from build123d import *

# Parameters (mm, degrees)
SKETCH1_R                        = 23.01875
SKETCH1_R_2                      = 11.1125
BOSS_EXTRUDE1_DEPTH              = 76.2
SKETCH2_R                        = 16.66875
SKETCH2_R_2                      = 11.1125
BOSS_EXTRUDE2_DEPTH              = 31.75
CUT_EXTRUDE1_DEPTH               = 44.45
F_10_0_1935_DIAMETER_HOLE1_D     = 4.9149
F_10_0_1935_DIAMETER_HOLE1_DEPTH = 3.175
F_10_0_1935_DIAMETER_HOLE1_TIP   = 1.476584928


with BuildPart() as part:
    # Sketch1 → Boss-Extrude1 (new body)
    with BuildSketch(Plane(origin=(0, 0, 0), x_dir=(1, 0, 0), z_dir=(0, 1, 0))):
        Circle(SKETCH1_R)
        Circle(SKETCH1_R_2, mode=Mode.SUBTRACT)
    extrude(amount=BOSS_EXTRUDE1_DEPTH)

    # Sketch2 → Boss-Extrude2 (add)
    with BuildSketch(Plane(origin=(0, 76.2, 0), x_dir=(1, 0, 0), z_dir=(0, 1, 0))):
        Circle(SKETCH2_R)
        Circle(SKETCH2_R_2, mode=Mode.SUBTRACT)
    extrude(amount=BOSS_EXTRUDE2_DEPTH)

    # Sketch3 → Cut-Revolve1 (revolve, cut)
    with BuildSketch(Plane(origin=(0, 0, 0), x_dir=(0, 0, -1), z_dir=(1, 0, 0))):
        Polygon((16.66875, 107.95), (16.66875, 100.57660721), (11.1125, 107.95), align=None)
    revolve(axis=Axis((0, 107.95, 0), (0, 1, 0)), mode=Mode.SUBTRACT)

    # Sketch4 → Cut-Extrude1 (cut)
    with BuildSketch(Plane(origin=(0, 76.2, 0), x_dir=(1, 0, 0), z_dir=(0, 1, 0))):
        with BuildLine():
            Line((8.400260413, -21.43125), (-8.400260413, -21.43125))
            ThreePointArc((-8.400260413, -21.43125), (0, -23.01875), (8.400260413, -21.43125))
        make_face()
    extrude(amount=-CUT_EXTRUDE1_DEPTH, mode=Mode.SUBTRACT)

    # Sketch8 → Cut-Revolve4 (revolve, cut)
    with BuildSketch(Plane.XY):
        with BuildLine():
            Line((0, 0), (-3.369464108, 0))
            ThreePointArc((-3.369464108, 0), (-13.321537524, 0.798864496), (-23.01875, 3.175))
            Line((-23.01875, 3.175), (-23.01875, -4.469484217))
            Line((-23.01875, -4.469484217), (0, -4.469484217))
            Line((0, -4.469484217), (0, 0))
        make_face()
    revolve(axis=Axis((0, 0, 0), (0, 1, 0)), mode=Mode.SUBTRACT)

    # 10 _0.1935_ Diameter Hole1
    with Locations(Plane.XY.offset(21.43125)):
        with Locations((0, 68.2625), (0, 39.6875)):
            Hole(F_10_0_1935_DIAMETER_HOLE1_D / 2, depth=F_10_0_1935_DIAMETER_HOLE1_DEPTH)
            with Locations((0, 0, -(F_10_0_1935_DIAMETER_HOLE1_DEPTH + F_10_0_1935_DIAMETER_HOLE1_TIP / 2))):  # 118° drill point
                Cone(0, F_10_0_1935_DIAMETER_HOLE1_D / 2, F_10_0_1935_DIAMETER_HOLE1_TIP, mode=Mode.SUBTRACT)


solid = part.part
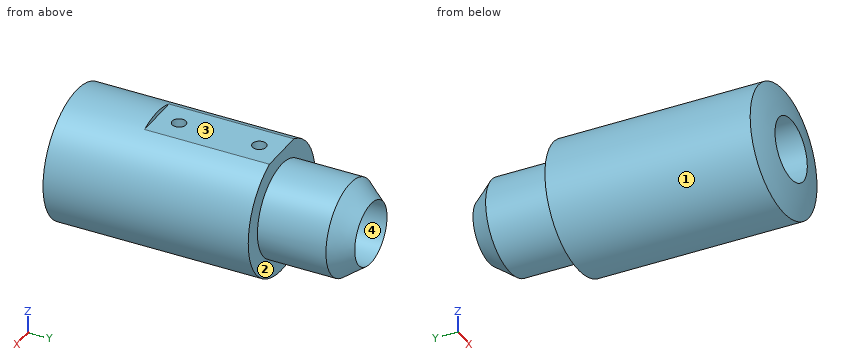
Can you work these out from the model? Positions are in its coordinate system, mm. Face numbers are marked on the shaded views. Give positions to 0.01 mm unless a question says otherwise; leave off trailing zeros. Loops run counter-clockwise (first coordinate to the right, second up) from the corner with the lowest first, then second, coordinate; pieces in that order, holes last. Notation, with made-up numbers: M 59.25,10.5 L 107.25,10.5 A12 cw 107.25,30.5 Z; hole C -29,-21.5 d2. An arc over 180 degrees is marked long. One line per item, written item: value. Start each with the question number.
1) If we section it at C-C, the plane y = 97: Write out the boundary of the cut face in (x, z) (1 decimal).
2) Thinking about a two-plate mould opening in Z: for the marked faces 1, 2, 3 and 4, which applies, +Z half, -Z half, draft (parallel to the pull), parting line (faces both ways), or undercut?
3) If I drill on line 1 (Y direction, x = 0, z = 20.35); line 2 (Y direction, x = 0, z = 20); line 3 (Z direction, x = 0, y = 48), over which ranges is the centre line in solid material (lowest first)? Write a range as [from, to].
4) If we section it at A-A, the plane y = 46.5: Write out the boundary of the cut face in (x, z) (1 decimal), and give its area (3 significant figures).
5) I'm going to push flat-ended pins straight in: pin 1 (13.5 mm diameter, centred on x = -11, z = -2.5, fed in from +Y); pin 2 (8 mm diameter, centred on y = 81.5, z = -2.5, fed in from +X); pin 3 (3 mm diameter, centred on x = -9.5, y = 50, fed in from -Z); pin 4 (2 mm diameter, centred on x = 3.5, z = -17, fed in from -Y). Where does each tip first touch, or does it pass through?
6) If we section it at B-B, the plane y = 11: Write out the boundary of the cut face in (x, z) (1 decimal).
Completed:
1. outline: C 0,0 d33.3; hole C 0,0 d22.2
2. face 1: parting line
2. face 2: draft
2. face 3: +Z half
2. face 4: undercut
3. line 1: y = [2.36, 37.23], [42.14, 65.81], [70.72, 76.2]
3. line 2: y = [2.26, 37.23], [42.14, 65.81], [70.72, 76.2]
3. line 3: z = [-23.02, -11.11], [11.11, 21.43]
4. outline: M -8.4,21.4 A23 ccw long 8.4,21.4 Z; hole C 0,0 d22.2
4. area: 1,260 mm^2
5. pin 1: stops at y = 107.95
5. pin 2: stops at x = 16.67
5. pin 3: stops at z = -21.58
5. pin 4: stops at y = 1.37
6. outline: C 0,0 d46; hole C 0,0 d22.2
